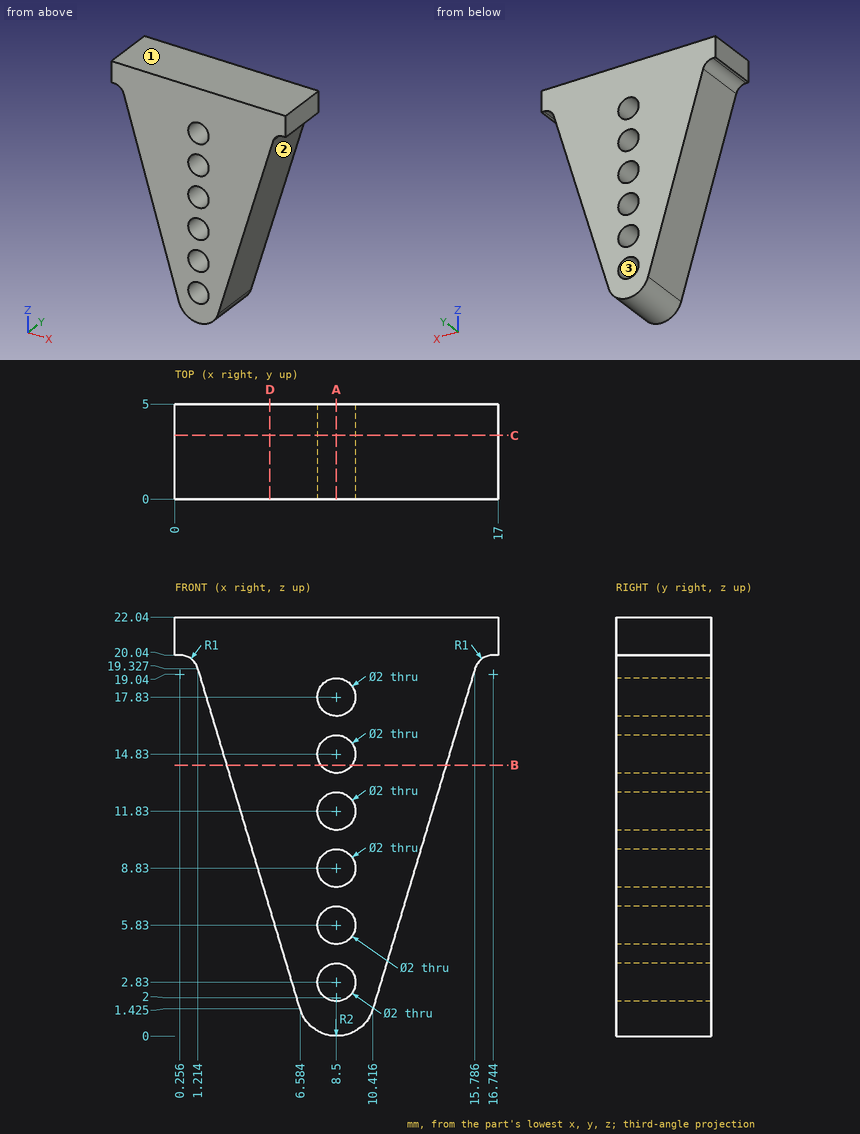
Design review of the part shown in the three views and the two pictorial views. Dimensions are in mm from the part's minimum x, y and z. Coordinates: 2 decimals unless noted, no trailing zeros. Loops run counter-clockwise (first coordinate to the right, second up) from the corner with the lowest first, then second, coordinate; pieces in that order, holes last.
Q1. We need section A-A on x = 8.5. State the section outline as (y, z) points.
Reported:
outline: (0, 0) - (5, 0) - (5, 1.83) - (0, 1.83) - close; (0, 3.83) - (5, 3.83) - (5, 4.83) - (0, 4.83) - close; (0, 6.83) - (5, 6.83) - (5, 7.83) - (0, 7.83) - close; (0, 9.83) - (5, 9.83) - (5, 10.83) - (0, 10.83) - close; (0, 12.83) - (5, 12.83) - (5, 13.83) - (0, 13.83) - close; (0, 15.83) - (5, 15.83) - (5, 16.83) - (0, 16.83) - close; (0, 18.83) - (5, 18.83) - (5, 22.04) - (0, 22.04) - close
Q2. To check wall thickness, follow line 1 (X direction, y = 4.6, z = 5); line 2 (X direction, y = 1.2, z = 18.25); line 3 (X direction, y = 1.6, z = 13.5). State the ranges of each line that lie inside material, in increasing order.
Reported:
line 1: x = 5.51 to 7.94, 9.06 to 11.49
line 2: x = 1.54 to 7.59, 9.41 to 15.46
line 3: x = 2.96 to 14.04
Q3. The part is to be moulded in two halves that separate along X. For the marked faces 1, 2 and 3, say which applies: +X half, -X half, draft (parallel to the pull), parting line (faces both ways), or undercut.
Reported:
face 1: draft
face 2: +X half
face 3: undercut
Q4. We need section C-C on y = 3.35. State how many separate pieces and enclosed holes the cut face has, and give its area (3 significant figures).
Reported:
separate pieces: 1
enclosed holes: 6
area: 195 mm2
Q5. We need section D-D on x = 5. State the section outline as (y, z) points.
Reported:
outline: (0, 6.71) - (5, 6.71) - (5, 22.04) - (0, 22.04) - close
Q6. For pin 1 (2 mm diameter, centred on y = 1, z = 13.5, fed in from +X); pin 2 (1.5 mm diameter, centred on y = 3.5, z = 5, fed in from +X), all flat-tipped, find the tip position at first contact; note any pin that passes through.
Reported:
pin 1: stops at x = 14.34
pin 2: stops at x = 11.71
Q7. We need section B-B on z = 14.25. State the section outline as (x, y) points (1 decimal), and give its area (3 significant figures).
Reported:
outline: (2.7, 0) - (7.7, 0) - (7.7, 5) - (2.7, 5) - close; (9.3, 0) - (14.3, 0) - (14.3, 5) - (9.3, 5) - close
area: 49.5 mm2
